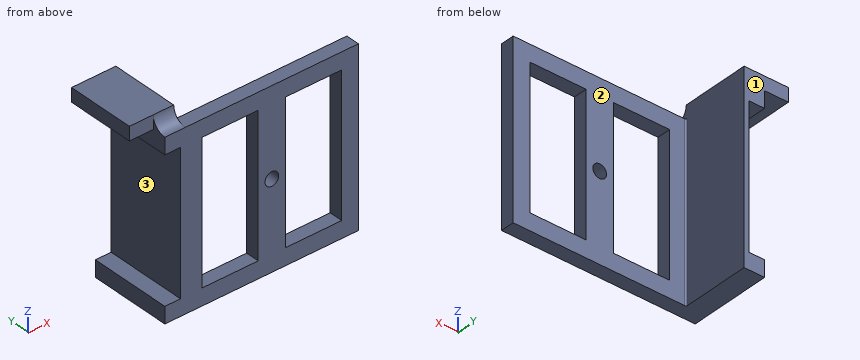
from build123d import *

# Parameters (mm, degrees)
SKETCH2_R               = 1
SKETCH2_W               = 8.25
SKETCH2_H               = 20.5
BOSS_EXTRUDE1_DEPTH     = 2
SKETCH3_W               = 3
SKETCH3_H               = 25.4
BOSS_EXTRUDE2_DEPTH     = 10
FILLET1_R               = 0.25
SKETCH5_W               = 6.5
SKETCH5_H               = 10
BOSS_EXTRUDE3_DEPTH     = 2
CUT_EXTRUDE1_DEPTH      = 27.994999537
CUT_EXTRUDE1_DEPTH_BACK = 27.994999537
SKETCH6_W               = 2.6
SKETCH6_H               = 20.6
FILLET3_R               = 2


with BuildPart() as part:
    # Sketch2 → Boss-Extrude1 (new body)
    with BuildSketch(Plane(origin=(0, 0, 0), x_dir=(1, 0, 0), z_dir=(0, 1, 0))):
        Polygon((-12.7, 12.7), (-15.7, 12.7), (-15.7, -12.7), (-12.7, -12.7), (12.7, -12.7), (12.7, 12.7), align=None)
        with Locations(Location((0, 0, 0), (0, 0, 270))):
            Circle(SKETCH2_R, mode=Mode.SUBTRACT)
        with Locations((6.125, 0)):
            Rectangle(SKETCH2_W, SKETCH2_H, mode=Mode.SUBTRACT)
        with Locations((-6.125, 0)):
            Rectangle(SKETCH2_W, SKETCH2_H, mode=Mode.SUBTRACT)
    extrude(amount=BOSS_EXTRUDE1_DEPTH)

    # Sketch3 → Boss-Extrude2 (add)
    with BuildSketch(Plane(origin=(0, 2, 0), x_dir=(1, 0, 0), z_dir=(0, 1, 0))):
        with Locations((-14.2, 0)):
            Rectangle(SKETCH3_W, SKETCH3_H)
    extrude(amount=BOSS_EXTRUDE2_DEPTH)

    # Fillet1
    fillet1_edges = [part.edges().sort_by_distance(p)[0] for p in [
        (-12.7, 2, 0),
    ]]
    fillet(fillet1_edges, radius=FILLET1_R)

    # Sketch5 → Boss-Extrude3 (add)
    with BuildSketch(Plane.XY.offset(12.7)):
        with Locations((-15.95, 7)):
            Rectangle(SKETCH5_W, SKETCH5_H)
    extrude(amount=BOSS_EXTRUDE3_DEPTH)

    # Sketch6 → Cut-Extrude1 (cut, two sides: drawn at the far end of the back side and taken through both)
    with BuildSketch(Plane.XZ.offset(-CUT_EXTRUDE1_DEPTH_BACK)):
        with Locations((-14.7, 0)):
            Rectangle(SKETCH6_W, SKETCH6_H)
    extrude(amount=CUT_EXTRUDE1_DEPTH + CUT_EXTRUDE1_DEPTH_BACK, mode=Mode.SUBTRACT)

    # Fillet3
    fillet3_edges = [part.edges().sort_by_distance(p)[0] for p in [
        (-14.2, 2, 12.7),
    ]]
    fillet(fillet3_edges, radius=FILLET3_R - 0.0001)  # a hair under: the kernel refuses the full size


solid = part.part
Build history of the part. All positions in model axes, mm. Face numbers are marked on the shaded views. A direction names the side the tool comes from. Round coordinates to 2 decimals unless told otherwise and drop trailing zeros. Write each loop counter-clockwise with the first axis right and the second up, starting at its lowest first coordinate (ties: lowest second). Pieces come first, ordered by that corner, then holes. Notation, with made-up numbers: M 30,-5.5 L 75,-5.5 A23 ccw 75,33.5 Z; hole C -10,-6 d6. An arc over 180 degrees is marked long. Answer in a Markdown table with one row per item.
1. Probe L1, parallel to X at y = 1.25, z = 0; L2, parallel to X at y = 1.5, z = 4; L3, parallel to Z at x = -15, y = 10.5. List the from-to ranges inside material, lowest first. Write a range as [from, to].
Geometry check:
| item | result |
|---|---|
| L1 | [-13.4, -10.25], [-2, -1], [1, 2], [10.25, 12.7] |
| L2 | [-13.4, -10.25], [-2, 2], [10.25, 12.7] |
| L3 | [-12.7, -10.3], [10.3, 14.7] |
2. Saw through at C-C (y = 6). List the corners of the cut face in (x, z), and give its area (3 significant figures).
Geometry check:
| item | result |
|---|---|
| outline | M -19.2,12.7 L -15.7,12.7 L -15.7,10.3 L -13.4,10.3 L -13.4,-10.3 L -15.7,-10.3 L -15.7,-12.7 L -12.7,-12.7 L -12.7,14.7 L -19.2,14.7 Z |
| area | 41.8 mm2 |
3. Saw through at A-A (x = -9). List the corners of the cut face in (y, z), and give its area (3 significant figures).
Geometry check:
| item | result |
|---|---|
| outline | M 0,-12.7 L 2,-12.7 L 2,-10.25 L 0,-10.25 Z; M 0,10.25 L 2,10.25 L 2,12.7 L 0,12.7 Z |
| area | 9.80 mm2 |
4. Flat gauge pins, fed straight in: P1, Ø6, axis at x = 1, y = 4, coming from the +Z side; P2, Ø2, axis at x = -17, z = 14, coming from the -Y side; P3, Ø1.8, axis at x = -17, y = 7.5, coming from the -Z side. Where does each tip first touch, or does it go through?
Geometry check:
| item | result |
|---|---|
| P1 | z = 12.7 |
| P2 | y = 2 |
| P3 | z = 12.7 |
5. Saw through at D-D (z = 7.75). List the corners of the cut face in (x, y), and give its area (3 significant figures).
Geometry check:
| item | result |
|---|---|
| outline | M -13.4,0 L -10.25,0 L -10.25,2 L -12.45,2 A0.25 cw -12.7,2.25 L -12.7,12 L -13.4,12 Z; M -2,0 L 2,0 L 2,2 L -2,2 Z; M 10.25,0 L 12.7,0 L 12.7,2 L 10.25,2 Z |
| area | 26.2 mm2 |
6. Which spindle directions (+Z, -Z, +X, -X, +Y, -Y) get a long thin tool onto all of the face, cutting with end or side? Do the marked faces 1, 2 and 3. Say none if no direction does.
Geometry check:
| item | result |
|---|---|
| face 1 | +Z, -Z, +X, -X, +Y |
| face 2 | +Z, -Z, +X, +Y |
| face 3 | -X, +Y, -Y |
7. Saw through at B-B (z = 0). List the corners of the cut face in (x, y), and give its area (3 significant figures).
Geometry check:
| item | result |
|---|---|
| outline | M -13.4,0 L -10.25,0 L -10.25,2 L -12.45,2 A0.25 cw -12.7,2.25 L -12.7,12 L -13.4,12 Z; M -2,0 L -1,0 L -1,2 L -2,2 Z; M 1,0 L 2,0 L 2,2 L 1,2 Z; M 10.25,0 L 12.7,0 L 12.7,2 L 10.25,2 Z |
| area | 22.2 mm2 |
